Work out the finished part from the listing and answer in its coordinate system (mm). A direction names the side the tool comes from. Give positions to 0.01 mm unless a question says otherwise; leave off trailing zeros. Loops run counter-clockwise (first coordinate to the right, second up) from the corner with the lowest first, then second, coordinate; pieces in that order, holes last. Notation, with made-up numbers: (-14.75, 3) -> (44.25, 3) arc R33 ccw to (44.25, 34) -> close; hole circle Ø11 at (-3, 38). An arc over 180 degrees is marked (long way). Answer as CSV lines item,"result". Start each with the question number.
1. Flat-ended cylindrical pins translate along their axes: pin 1 Ø1.6 at (x, z) = (5, 1.5) entering from -Y; pin 2 Ø1 at (y, z) = (-5, -4.5) entering from +X; pin 3 Ø0.6 at (x, z) = (-5, -2) entering from -Y; pin 4 Ø5 at (y, z) = (-1, -4) entering from -X. Find the tip coordinate at first contact, or state that the pin passes through.
2. Determine the mould class of faces 4 (the face through (1, -5, -12)), 5 (the face through (0, 5.969, 0)), 6 (the face through (-1.54, -3.69, 0.16)), 7 (the face through (-7.493, 0.33, -9.859)) for opening direction X: +X half, -X half, draft (parallel to the pull), parting line (faces both ways), or undercut.
3. Find the intervals of material crossed by line 1 along X through (y, z) = (3.5, -4.5); line 2 along Y through (x, z) = (-4, -7.25); line 3 along Y through (x, z) = (3.25, -5.25), in increasing order.
4. Find section A-A, the plane y = 0. Give the vertices of the cut face in (x, z).
5. A tool of negligible diameter and unlimited length cuts with its end or side. For faces 1 (the face through (-5, -0.5, 0)), 2 (the face through (3.936, 1.612, 11.754)), 3 (the face through (-3.92, 1.64, -11.75)), from which of +Z, -Z, +X, -X, +Y, -Y can it reach the whole face along a straight path? Write none if from no direction.
from build123d import *

# Parameters (mm, degrees)
ESQUISSE1_R        = 7.5
BOSS_EXTRU_1_DEPTH = 12
ESQUISSE2_W        = 1.1
ESQUISSE2_H        = 0.35
CHANFREIN1_SIZE    = 1
CHANFREIN1_SIZE2   = 0.5
CHANFREIN2_SIZE    = 0.5
CHANFREIN2_SIZE2   = 1
CHANFREIN3_SIZE    = 0.5


with BuildPart() as part:
    # Esquisse1 → Boss.-Extru.1 (new, symmetric)
    with BuildSketch(Plane.XY):
        Circle(ESQUISSE1_R)
        with BuildLine():
            Line((3.866903212, 4.574009993), (2.452689649, 3.159796431))
            ThreePointArc((2.452689649, 3.159796431), (1.530733729, 3.69551813), (0.5, 3.968626967))
            Line((0.5, 3.968626967), (0.5, 5.968626967))
            Line((0.5, 5.968626967), (-0.5, 5.968626967))
            Line((-0.5, 5.968626967), (-0.5, 3.968626967))
            ThreePointArc((-0.5, 3.968626967), (-1.530733729, 3.69551813), (-2.452689649, 3.159796431))
            Line((-2.452689649, 3.159796431), (-3.866903212, 4.574009993))
            Line((-3.866903212, 4.574009993), (-4.574009993, 3.866903212))
            Line((-4.574009993, 3.866903212), (-3.159796431, 2.452689649))
            ThreePointArc((-3.159796431, 2.452689649), (-3.69551813, 1.530733729), (-3.968626967, 0.5))
            Line((-3.968626967, 0.5), (-5.968626967, 0.5))
            Line((-5.968626967, 0.5), (-5.968626967, -0.5))
            Line((-5.968626967, -0.5), (-3.968626967, -0.5))
            ThreePointArc((-3.968626967, -0.5), (-3.69551813, -1.530733729), (-3.159796431, -2.452689649))
            Line((-3.159796431, -2.452689649), (-4.574009993, -3.866903212))
            Line((-4.574009993, -3.866903212), (-3.866903212, -4.574009993))
            Line((-3.866903212, -4.574009993), (-2.452689649, -3.159796431))
            ThreePointArc((-2.452689649, -3.159796431), (-1.530733729, -3.69551813), (-0.5, -3.968626967))
            Line((-0.5, -3.968626967), (-0.5, -5.968626967))
            Line((-0.5, -5.968626967), (0.5, -5.968626967))
            Line((0.5, -5.968626967), (0.5, -3.968626967))
            ThreePointArc((0.5, -3.968626967), (1.530733729, -3.69551813), (2.452689649, -3.159796431))
            Line((2.452689649, -3.159796431), (3.866903212, -4.574009993))
            Line((3.866903212, -4.574009993), (4.574009993, -3.866903212))
            Line((4.574009993, -3.866903212), (3.159796431, -2.452689649))
            ThreePointArc((3.159796431, -2.452689649), (3.69551813, -1.530733729), (3.968626967, -0.5))
            Line((3.968626967, -0.5), (5.968626967, -0.5))
            Line((5.968626967, -0.5), (5.968626967, 0.5))
            Line((5.968626967, 0.5), (3.968626967, 0.5))
            ThreePointArc((3.968626967, 0.5), (3.69551813, 1.530733729), (3.159796431, 2.452689649))
            Line((3.159796431, 2.452689649), (4.574009993, 3.866903212))
            Line((4.574009993, 3.866903212), (3.866903212, 4.574009993))
        make_face(mode=Mode.SUBTRACT)
    extrude(amount=BOSS_EXTRU_1_DEPTH, both=True)

    # Esquisse2 → Enlèvement de matière-Révolution1 (revolve, cut)
    with BuildSketch(Plane(origin=(0, 0, 0), x_dir=(0, 0, -1), z_dir=(1, 0, 0)), mode=Mode.PRIVATE) as enl_vement_de_mati_re_r_volution1_sk:
        with Locations((-8.2, 7.325)):
            Rectangle(ESQUISSE2_W, ESQUISSE2_H)
        with Locations((8.2, 7.325)):
            Rectangle(ESQUISSE2_W, ESQUISSE2_H)
    revolve(enl_vement_de_mati_re_r_volution1_sk.sketch.rotate(Axis((0, 0, 12), (0, 0, -1)), 90), axis=Axis((0, 0, 12), (0, 0, -1)), mode=Mode.SUBTRACT)

    # Chanfrein1
    chanfrein1_edges = [part.edges().sort_by_distance(p)[0] for p in [
        (-7.5, 0, 12),
    ]]
    chanfrein1_side = [part.faces().sort_by_distance(p)[0] for p in [
        (-7.5, 0, 10.375),
    ]]
    chamfer(chanfrein1_edges, length=CHANFREIN1_SIZE, length2=CHANFREIN1_SIZE2, reference=chanfrein1_side[0])

    # Chanfrein2
    chanfrein2_edges = [part.edges().sort_by_distance(p)[0] for p in [
        (-7.5, 0, -12),
    ]]
    chanfrein2_side = [part.faces().sort_by_distance(p)[0] for p in [
        (-7.287867966, 0, -12),
    ]]
    chamfer(chanfrein2_edges, length=CHANFREIN2_SIZE, length2=CHANFREIN2_SIZE2, reference=chanfrein2_side[0])

    # Chanfrein3
    chanfrein3_edges = [part.edges().sort_by_distance(p)[0] for p in [
        (-1.530733729, 3.69551813, -12),
        (-3.69551813, 1.530733729, -12),
        (-3.69551813, -1.530733729, -12),
        (-1.530733729, -3.69551813, -12),
        (1.530733729, -3.69551813, -12),
        (3.69551813, -1.530733729, -12),
        (3.69551813, 1.530733729, -12),
        (1.530733729, 3.69551813, -12),
        (-1.530733729, 3.69551813, 12),
        (-3.69551813, 1.530733729, 12),
        (-3.69551813, -1.530733729, 12),
        (-1.530733729, -3.69551813, 12),
        (1.530733729, -3.69551813, 12),
        (3.69551813, -1.530733729, 12),
        (3.69551813, 1.530733729, 12),
        (1.530733729, 3.69551813, 12),
    ]]
    chamfer(chanfrein3_edges, length=CHANFREIN3_SIZE)


solid = part.part
Resolved:
1,pin 1,"stops at y = -6.21"
1,pin 2,"stops at x = 6"
1,pin 3,"stops at y = -5.84"
1,pin 4,"stops at x = -7.5"
2,face 4,"draft"
2,face 5,"undercut"
2,face 6,"undercut"
2,face 7,"parting line"
3,line 1,"x = -6.63 to -4.21, -2.79 to -1.94, 1.94 to 2.79, 4.21 to 6.63"
3,line 2,"y = -6.34 to -4.44, -3.29 to -0.5, 0.5 to 3.29, 4.44 to 6.34"
3,line 3,"y = -6.76 to -3.96, -2.54 to -2.33, 2.33 to 2.54, 3.96 to 6.76"
4,outline,"(-7.5, -11) -> (-7, -12) -> (-5.97, -12) -> (-5.97, 12) -> (-7, 12) -> (-7.5, 11) -> (-7.5, 8.75) -> (-7.15, 8.75) -> (-7.15, 7.65) -> (-7.5, 7.65) -> (-7.5, -7.65) -> (-7.15, -7.65) -> (-7.15, -8.75) -> (-7.5, -8.75) -> close; (5.97, -12) -> (7, -12) -> (7.5, -11) -> (7.5, -8.75) -> (7.15, -8.75) -> (7.15, -7.65) -> (7.5, -7.65) -> (7.5, 7.65) -> (7.15, 7.65) -> (7.15, 8.75) -> (7.5, 8.75) -> (7.5, 11) -> (7, 12) -> (5.97, 12) -> close"
5,face 1,"+Z, -Z"
5,face 2,"+Z"
5,face 3,"-Z"
